Here's how the part is built. I have some questions about the finished solid (model axes, mm). A direction names the side the tool comes from. Coordinates: 2 decimals unless noted, no trailing zeros. Write each loop counter-clockwise with the first axis right and the second up, starting at its lowest first coordinate (ties: lowest second). Pieces come first, ordered by that corner, then holes.
Item 1: I'm going to push flat-ended pins straight in: pin 1 Ø3 at (x, z) = (1, 6) entering from +Y; pin 2 Ø1 at (x, z) = (-3, 5) entering from -Y; pin 3 Ø3.5 at (x, y) = (0.5, 0) entering from -Z. Where does each tip first touch, or does it pass through?
Item 2: If we section it at C-C (z = 6.25): Please give me the cut outline in (x, y).
Item 3: If we section it at A-A (x = 0): Please give me the cut outline in (y, z), then the cut area to 3 significant figures.
Item 4: If we section it at B-B (z = 2): Please give me the cut outline in (x, y), then the cut area to 3 significant figures.
Item 5: If I drill on line 1 (Y direction, x = -1.75, z = 2); line 2 (Y direction, x = 0, z = 5.45); line 3 (Z direction, x = 4, y = -4.5), over which ranges is the centre line in solid material (lowest first)?
Item 6: For faces 1 (the face through (3, 2, 2)), 2 (the face through (0, -4.95, 2)), 3 (the face through (-0.534, 4.065, 5.726)), which set-ups out of +Z, -Z, +X, -X, +Y, -Y let a thin tool reach every point of the face, with its end or its side?
from build123d import *

# Parameters (mm, degrees)
ESQUISSE1_W             = 9.9
ESQUISSE1_H             = 9.9
BOSS_EXTRU_1_DEPTH      = 4
ENL_V_MAT_EXTRU_1_DEPTH = 3.2
ESQUISSE4_R             = 4.1
BOSS_EXTRU_2_DEPTH      = 4
CHANFREIN1_SIZE         = 0.5
ESQUISSE5_R             = 2.2
ENL_V_MAT_EXTRU_3_DEPTH = 11.63038099
CHANFREIN2_SIZE         = 0.5


with BuildPart() as part:
    # Esquisse1 → Boss.-Extru.1 (new body)
    with BuildSketch(Plane.XY):
        Rectangle(ESQUISSE1_W, ESQUISSE1_H)
    extrude(amount=BOSS_EXTRU_1_DEPTH)

    # Esquisse2 → Enlèv. mat.-Extru.1 (cut)
    with BuildSketch(Plane.XY):
        Polygon((4.156921938, 0), (2.078460969, 3.6), (-2.078460969, 3.6), (-4.156921938, 0), (-2.078460969, -3.6), (2.078460969, -3.6), align=None)
    extrude(amount=ENL_V_MAT_EXTRU_1_DEPTH, mode=Mode.SUBTRACT)

    # Esquisse4 → Boss.-Extru.2 (add)
    with BuildSketch(Plane.XY.offset(4)):
        Circle(ESQUISSE4_R)
    extrude(amount=BOSS_EXTRU_2_DEPTH)

    # Chanfrein1
    chanfrein1_edges = [part.edges().sort_by_distance(p)[0] for p in [
        (-4.1, 0, 8),
    ]]
    chamfer(chanfrein1_edges, length=CHANFREIN1_SIZE)

    # Esquisse5 → Enlèv. mat.-Extru.3 (cut, through all)
    with BuildSketch(Plane.XY.offset(8)):
        Circle(ESQUISSE5_R)
    extrude(amount=-ENL_V_MAT_EXTRU_3_DEPTH, mode=Mode.SUBTRACT)

    # Chanfrein2
    chanfrein2_edges = [part.edges().sort_by_distance(p)[0] for p in [
        (4.95, -4.95, 2),
        (-4.95, -4.95, 2),
        (-4.95, 4.95, 2),
        (4.95, 4.95, 2),
    ]]
    chamfer(chanfrein2_edges, length=CHANFREIN2_SIZE)


solid = part.part
Answer list:
1. pin 1: stops at y = 4.1
1. pin 2: stops at y = -3.25
1. pin 3: stops at z = 3.2
2. outline: circle Ø8.2 at (0, 0); hole circle Ø4.4 at (0, 0)
3. outline: (-4.95, 0) - (-3.6, 0) - (-3.6, 3.2) - (-2.2, 3.2) - (-2.2, 8) - (-3.6, 8) - (-4.1, 7.5) - (-4.1, 4) - (-4.95, 4) - close; (2.2, 3.2) - (3.6, 3.2) - (3.6, 0) - (4.95, 0) - (4.95, 4) - (4.1, 4) - (4.1, 7.5) - (3.6, 8) - (2.2, 8) - close
3. area: 28.0 mm2
4. outline: (-4.95, -4.45) - (-4.45, -4.95) - (4.45, -4.95) - (4.95, -4.45) - (4.95, 4.45) - (4.45, 4.95) - (-4.45, 4.95) - (-4.95, 4.45) - close; hole (-4.16, 0) - (-2.08, -3.6) - (2.08, -3.6) - (4.16, 0) - (2.08, 3.6) - (-2.08, 3.6) - close
4. area: 52.6 mm2
5. line 1: y = -4.95 to -3.6, 3.6 to 4.95
5. line 2: y = -4.1 to -2.2, 2.2 to 4.1
5. line 3: z = 0 to 4
6. face 1: -Z
6. face 2: +Z, -Z, +X, -X, -Y
6. face 3: +Z
